Part print with two shaded views. Sizes in mm from the minimum x, y, z corner. A direction names the side the tool comes from. Round coordinates to 2 decimals unless told otherwise and drop trailing zeros. Loops run counter-clockwise (first coordinate to the right, second up) from the corner with the lowest first, then second, coordinate; pieces in that order, holes last. Notation, with made-up numbers: (70, -18.5) -> (88, -18.5) arc R21 ccw to (88, -13.5) -> close; hole circle Ø1 at (-4, -21.5). An arc over 180 degrees is marked (long way). Use a Markdown table: item, result. Add a question column.
Item 1: Flat gauge pins, fed straight in: pin 1 (10 mm diameter, centred on x = 10.5, z = 10, fed in from +Y); pin 2 (0.8 mm diameter, centred on x = 20.5, z = 17.5, fed in from +Y); pin 3 (5 mm diameter, centred on y = 58, z = 17.5, fed in from -X). Where does each tip first touch, or does it go through?
Item 2: Probe line 1 (Y direction, x = 8.5, z = 31); line 2 (X direction, y = 55, z = 20.5); line 3 (Z direction, x = 3, y = 32). List the from-to ranges inside material, lowest first. Write a range as [from, to].
Item 3: Cut at B-B, the plane z = 21. List the corners of the cut face in (x, y).
Item 4: Cut at C-C, the plane y = 45. List the corners of the cut face in (x, z).
Item 5: Cut at D-D, the plane x = 8. List the corners of the cut face in (y, z), plus the area to 3 significant figures.
Item 6: Which spindle directions (+Z, -Z, +X, -X, +Y, -Y) get a long thin tool onto all of the face, cutting with end or side? Do the marked faces 1 and 2. Say none if no direction does.
Item 7: Cut at A-A, the plane x = 21. List the corners of the cut face in (y, z).
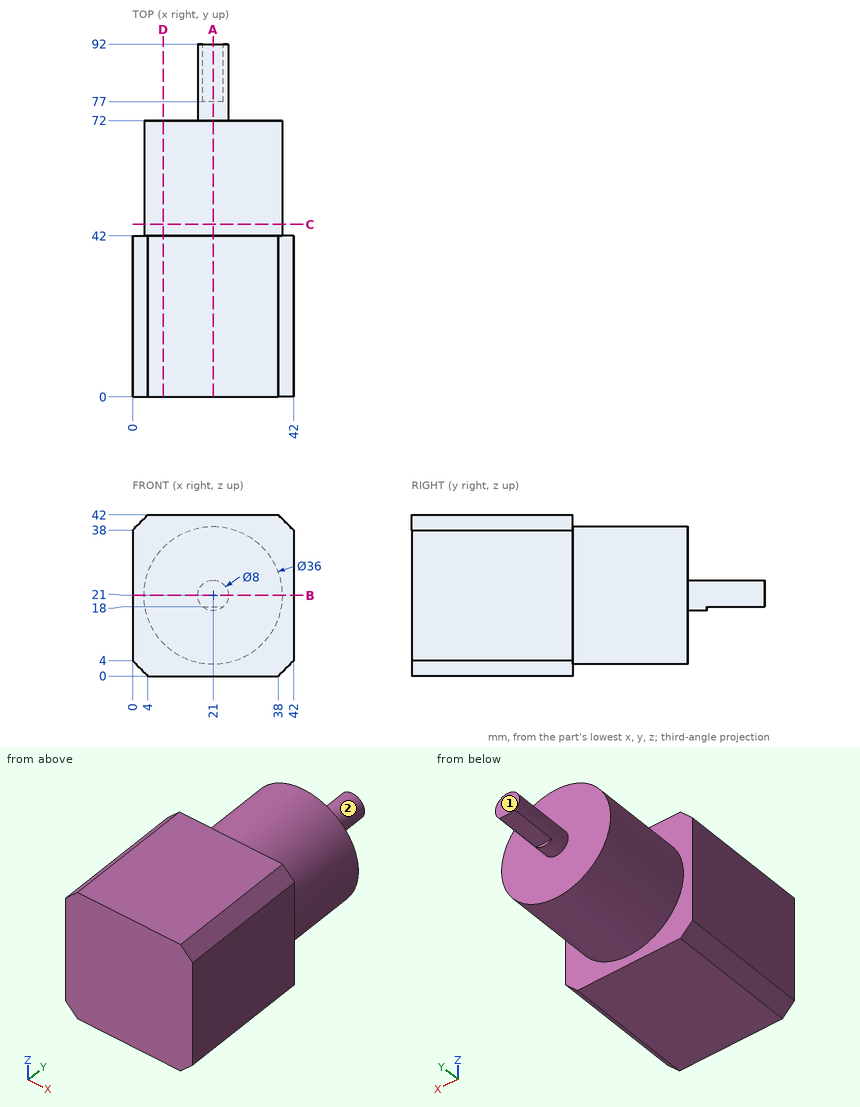
A:
| question | item | result |
|---|---|---|
| 1 | pin 1 | stops at y = 72 |
| 1 | pin 2 | stops at y = 77 |
| 1 | pin 3 | stops at x = 3.03 |
| 2 | line 1 | y = [0, 72] |
| 2 | line 2 | x = [3.01, 38.99] |
| 2 | line 3 | z = [1, 41] |
| 3 | outline | (0, 0) -> (42, 0) -> (42, 42) -> (39, 42) -> (39, 72) -> (25, 72) -> (25, 92) -> (17, 92) -> (17, 72) -> (3, 72) -> (3, 42) -> (0, 42) -> close |
| 4 | outline | circle Ø36 at (21, 21) |
| 5 | outline | (0, 0) -> (42, 0) -> (42, 8.55) -> (72, 8.55) -> (72, 33.45) -> (42, 33.45) -> (42, 42) -> (0, 42) -> close |
| 5 | area | 2,510 mm^2 |
| 6 | face 1 | +Z, -Z, +X, -X, +Y |
| 6 | face 2 | +Y |
| 7 | outline | (0, 0) -> (42, 0) -> (42, 3) -> (72, 3) -> (72, 17) -> (77, 17) -> (77, 18) -> (92, 18) -> (92, 25) -> (72, 25) -> (72, 39) -> (42, 39) -> (42, 42) -> (0, 42) -> close |
